Verification items for this drawing (mm, ordinates from the low corner). A direction names the side the tool comes from. Round coordinates to 2 decimals unless told otherwise and drop trailing zeros. Order: outer loops, then holes, each group sorted by start corner. A loop starts at its lowest first (then second) coordinate and runs counter-clockwise, first axis right, second up. Notation, with made-up numbers: (-33, 18) - (11, 18) arc R20 ccw to (11, 53) - close; hole circle Ø4 at (-18, 53.25). An arc over 180 degrees is marked (long way). One line per question, with ' | ' between items. Start each with the question number.
Q1. Sectioned sample at B-B, the plane y = 80. Enter the section's corners in (x, z) (3 decimals), then the cut area to 3 significant figures.
Q2. Sectioned sample at C-C, the plane z = 16.25. Enter the section's corners in (x, y) (3 decimals).
Q3. Gauge pin test, flat ends, axial feed: P1, Ø8, axis at y = 81, z = 16.5, coming from the +X side (3 decimals); P2, Ø4, axis at x = 12, z = 14.5, coming from the -Y side; P3, Ø12, axis at y = 88, z = 15.5, coming from the -X side. Record the tip position at first contact, or that the pin passes through.
Q4. Sectioned sample at D-D, the plane x = 7. Enter the section's corners in (y, z).
Q5. Material ranges on line 1 along Y through (x, z) = (15, 1.9) (3 decimals); line 2 along Z through (x, y) = (25.5, 66); line 3 along X through (y, z) = (82, 15.75), recorded low to high.
Q6. Sectioned sample at A-A, the plane x = 15. Enter the section's corners in (y, z) (3 decimals).
Q7. Tool access check on the marked faces 1 and 2. Record the directions out of +Z, -Z, +X, -X, +Y, -Y that give a thin tool (end or side, any length) a straight path to the whole face; none if there is none.
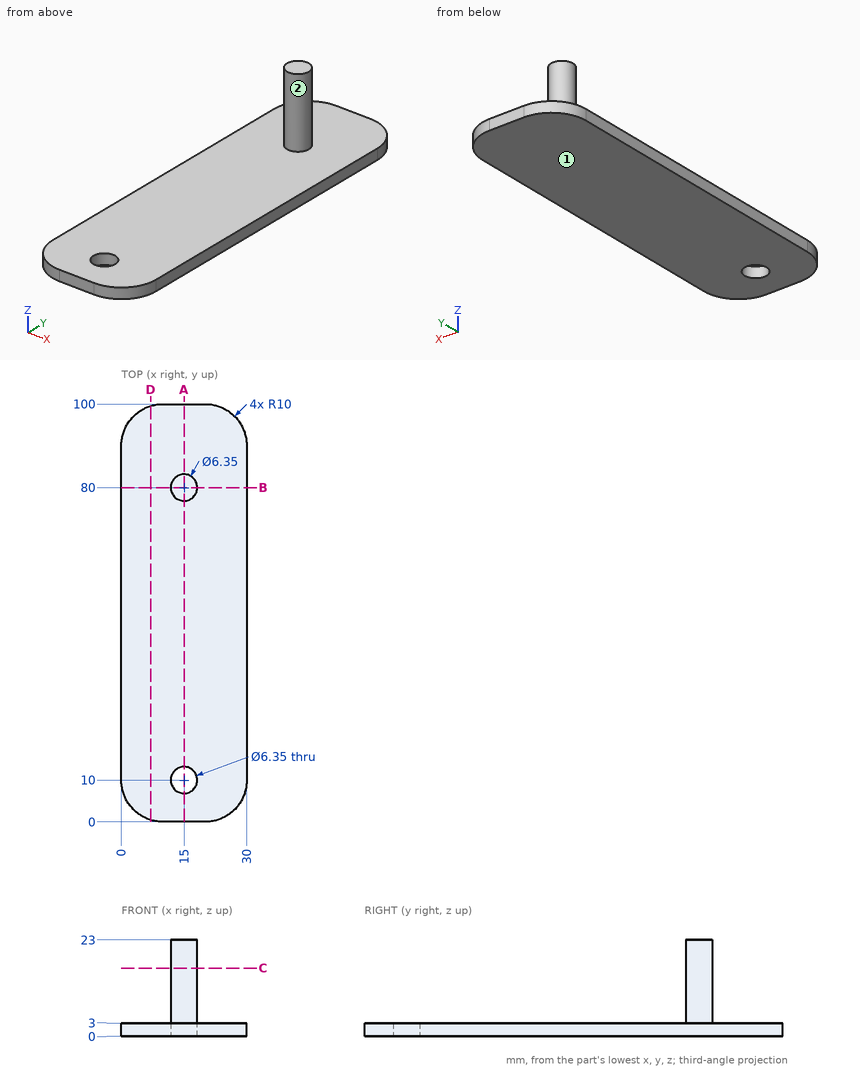
Determined:
1) outline: (0, 0) - (30, 0) - (30, 3) - (18.175, 3) - (18.175, 23) - (11.825, 23) - (11.825, 3) - (0, 3) - close | area: 217 mm2
2) outline: circle Ø6.35 at (15, 80)
3) P1: stops at x = 18.175 | P2: stops at y = 76.99 | P3: stops at x = 12.53
4) outline: (0.46, 0) - (99.54, 0) - (99.54, 3) - (0.46, 3) - close
5) line 1: y = 0 to 6.825, 13.175 to 100 | line 2: z = 0 to 3 | line 3: x = 12.53 to 17.47
6) outline: (0, 0) - (6.825, 0) - (6.825, 3) - (0, 3) - close; (13.175, 0) - (100, 0) - (100, 3) - (83.175, 3) - (83.175, 23) - (76.825, 23) - (76.825, 3) - (13.175, 3) - close
7) face 1: -Z, +X, -X, +Y, -Y | face 2: +Z
